Input: part model. Units: mm. Frame: model coordinates. Round coordinates to 2 decimals unless told otherwise and drop trailing zeros. Order: outer loops, then holes, each group sorted by start corner. A loop starts at its lowest first (then second) coordinate and runs counter-clockwise, first axis right, second up. Notation, with made-up numbers: (79, 64) -> (103, 64) arc R22 ccw to (103, 87) -> close; hole circle Ø1 at (-31.75, 49). An arc over 180 degrees is marked (long way). Use a Markdown table: item, result.
from build123d import *

# Parameters (mm, degrees)
SKETCH1_W                  = 127
SKETCH1_H                  = 101.6
BOSS_EXTRUDE1_DEPTH        = 6.35
F_9_0_196_DIAMETER_HOLE1_D = 4.9784
FILLET1_R                  = 12.7


with BuildPart() as part:
    # Sketch1 → Boss-Extrude1 (new body)
    with BuildSketch(Plane(origin=(0, 0, 0), x_dir=(0, 1, 0), z_dir=(0, 0, 1))):
        Rectangle(SKETCH1_W, SKETCH1_H)
    extrude(amount=BOSS_EXTRUDE1_DEPTH)

    # #9 (0.196) Diameter Hole1 (through all)
    with Locations(Plane.XY.offset(6.35)):
        with Locations((38.1, -50.8), (38.1, -25.4), (38.1, 25.4), (38.1, 50.8)):
            Hole(F_9_0_196_DIAMETER_HOLE1_D / 2)

    # Fillet1
    fillet1_edges = [part.edges().sort_by_distance(p)[0] for p in [
        (50.8, 63.5, 3.175),
        (50.8, -63.5, 3.175),
        (-50.8, -63.5, 3.175),
        (-50.8, 63.5, 3.175),
    ]]
    fillet(fillet1_edges, radius=FILLET1_R)


solid = part.part
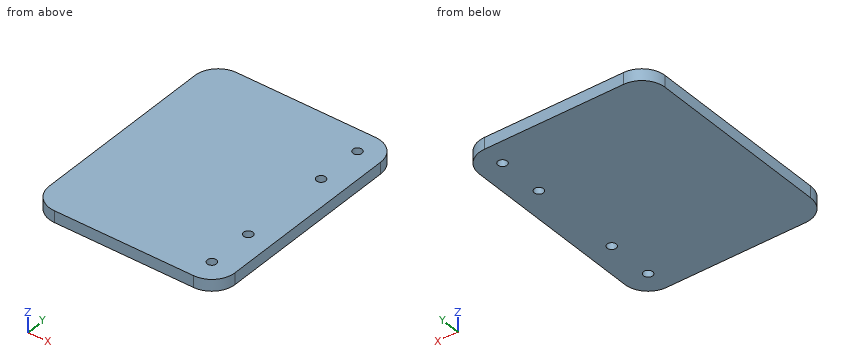
1) Line query: L1, parallel to Y at x = 38.1, z = 1.5; L2, parallel to Y at x = -38.5, z = 1; L3, parallel to X at y = 53, z = 4.75. Output: solid intervals per line, ascending. Write a range as [from, to].
Results found:
| item | result |
|---|---|
| L1 | y = [-63.5, -53.29], [-48.31, -27.89], [-22.91, 22.91], [27.89, 48.31], [53.29, 63.5] |
| L2 | y = [-63.49, 63.49] |
| L3 | x = [-50.61, 36.94], [39.26, 50.61] |
2) Cut plane A-A on y = -25.4. Return loops of the section in (x, z), and give its area (3 significant figures).
Results found:
| item | result |
|---|---|
| outline | (-50.8, 0) -> (35.61, 0) -> (35.61, 6.35) -> (-50.8, 6.35) -> close; (40.59, 0) -> (50.8, 0) -> (50.8, 6.35) -> (40.59, 6.35) -> close |
| area | 614 mm² |
3) Cut plane B-B on z = 3.25. Return loops of the section in (x, y), and give its area (3 significant figures).
Results found:
| item | result |
|---|---|
| outline | (-50.8, -50.8) arc R12.7 ccw to (-38.1, -63.5) -> (38.1, -63.5) arc R12.7 ccw to (50.8, -50.8) -> (50.8, 50.8) arc R12.7 ccw to (38.1, 63.5) -> (-38.1, 63.5) arc R12.7 ccw to (-50.8, 50.8) -> close; hole circle Ø4.98 at (38.1, -50.8); hole circle Ø4.98 at (38.1, -25.4); hole circle Ø4.98 at (38.1, 25.4); hole circle Ø4.98 at (38.1, 50.8) |
| area | 12,700 mm² |
4) Pin query (flat end, axial travel): pin 1 Ø2 at (x, y) = (-30.5, -49) entering from -Z; pin 2 Ø4.5 at (x, y) = (38.1, 25.4) entering from -Z. Return the tip coordinate at first contact, or that it passes through.
Results found:
| item | result |
|---|---|
| pin 1 | stops at z = 0 |
| pin 2 | passes through |
